Part model, mm, in its own coordinate system. A direction names the side the tool comes from. Give positions to 0.01 mm unless a question says otherwise; leave off trailing zeros. Loops run counter-clockwise (first coordinate to the right, second up) from the corner with the lowest first, then second, coordinate; pieces in that order, holes last. Notation, with made-up numbers: (48, 52) -> (59, 52) arc R25 cw to (59, 91) -> close; hole circle Ø4 at (25, 71). An arc over 180 degrees is marked (long way). One line per question, with ' | ' between items.
```python
from build123d import *

# Parameters (mm, degrees)
SKETCH1_R           = 3.935
EXTRUDE1_DEPTH      = 2
SKETCH2_R           = 2.7125
EXTRUDE2_DEPTH      = 1.4
SKETCH5_OUTSIDE_W   = 12.452
SKETCH5_OUTSIDE_H   = 12.452
SKETCH5_OUTSIDE_R   = 2.69
CUT_EXTRUDE1_DEPTH  = 0.35
CUT_EXTRUDE1_DRAFT  = 20
CHAMFER2_SIZE       = 0.127
SKETCH7_R           = 2
CUT_EXTRUDE3_DEPTH  = 7.521384056
BOSS_EXTRUDE1_DEPTH = 0.34
CIRPATTERN4_COUNT   = 30


with BuildPart() as part:
    # Sketch1 → Extrude1 (new body)
    with BuildSketch(Plane.XY):
        Circle(SKETCH1_R)
    extrude(amount=-EXTRUDE1_DEPTH)

    # Sketch2 → Extrude2 (add)
    with BuildSketch(Plane(origin=(0, 0, -2), x_dir=(-1, 0, 0), z_dir=(0, 0, -1))):
        with Locations(Location((0, 0, 0), (0, 0, 180))):
            Circle(SKETCH2_R)
    extrude(amount=EXTRUDE2_DEPTH)


with BuildPart() as cut_extrude1_tool:
    # Sketch5 outside → Cut-Extrude1 (with draft: the straight prism first)
    with BuildSketch(Plane(origin=(0, 0, -3.4), x_dir=(-1, 0, 0), z_dir=(0, 0, -1))):
        Rectangle(SKETCH5_OUTSIDE_W, SKETCH5_OUTSIDE_H)
        Circle(SKETCH5_OUTSIDE_R, mode=Mode.SUBTRACT)
    extrude(amount=-CUT_EXTRUDE1_DEPTH)
    # Cut-Extrude1: the draft: its side faces are tilted about the plane it starts from
    cut_extrude1_sides = [cut_extrude1_tool.faces().sort_by_distance(p)[0] for p in [
        (0, -6.226, -3.225),
        (-6.226, 0, -3.225),
        (0, 6.226, -3.225),
        (6.226, 0, -3.225),
        (2.69, 0, -3.225),
    ]]
    draft(cut_extrude1_sides, Plane(origin=(0, 0, -3.4), x_dir=(-1, 0, 0), z_dir=(0, 0, -1)), CUT_EXTRUDE1_DRAFT)


with BuildPart() as part_1:
    add(part.part)

    # Cut-Extrude1: cut by cut_extrude1_tool
    add(cut_extrude1_tool.part, mode=Mode.SUBTRACT)

    # Chamfer2
    chamfer2_edges = [part_1.edges().sort_by_distance(p)[0] for p in [
        (-3.935, 0, 0),
        (-3.935, 0, -2),
    ]]
    chamfer(chamfer2_edges, length=CHAMFER2_SIZE)

    # Sketch7 → Cut-Extrude3 (cut, through all)
    with BuildSketch(Plane.XY):
        Circle(SKETCH7_R)
    extrude(amount=-CUT_EXTRUDE3_DEPTH, mode=Mode.SUBTRACT)

    # Cut-Extrude6 cone 1 section (on through the dimple's axis) → Cut-Extrude6 (revolve, cut)
    with BuildSketch(Plane(origin=(0, 0, 0), x_dir=(0, -1, 0), z_dir=(1, 0, 0))):
        Polygon((0, 0), (2.0508, 0), (0, 2.0508), align=None)
    revolve(axis=Axis((0, 0, 0), (0, 0, -1)), mode=Mode.SUBTRACT)

    # Cut-Extrude7 cone 1 section (on through the dimple's axis) → Cut-Extrude7 (revolve, cut)
    with BuildSketch(Plane(origin=(0, 0, -3.4), x_dir=(0, 1, 0), z_dir=(1, 0, 0))):
        Polygon((0, 0), (2.0635, 0), (0, 2.0635), align=None)
    revolve(axis=Axis((0, 0, -3.4), (0, 0, 1)), mode=Mode.SUBTRACT)

    # Sketch16 → Boss-Extrude1 (add)
    with BuildSketch(Plane(origin=(0, 0, -2), x_dir=(-1, 0, 0), z_dir=(0, 0, -1))):
        with BuildLine():
            Line((0, 3.249), (-0.602777778, 2.644676767))
            ThreePointArc((-0.602777778, 2.644676767), (0, 2.7125), (0.602777778, 2.644676767))
            Line((0.602777778, 2.644676767), (0, 3.249))
        make_face()
    boss_extrude1 = extrude(amount=BOSS_EXTRUDE1_DEPTH)

    # CirPattern4: Boss-Extrude1 ×30 about axis
    cirpattern4_axis = Axis((0, 0, 0), (0, 0, 1))
    for i in range(1, CIRPATTERN4_COUNT):
        add(boss_extrude1.rotate(cirpattern4_axis, i * 360 / CIRPATTERN4_COUNT))


solid = part_1.part
```
1) Drill centre lines: line 1 (Y direction, x = 0, z = -0.9) (3 decimals); line 2 (Y direction, x = 0, z = -2.7); line 3 (Z direction, x = 3.25, y = -0.25). Where is each one in solid material? Low to high.
Found:
line 1: -3.935 to -2, 2 to 3.935 | line 2: -2.71 to -2, 2 to 2.71 | line 3: -2 to 0
2) Saw through at A-A (z = -2.7). Give the cut face in (x, y) (1 decimal), and give its area (3 significant figures).
Found:
outline: circle Ø5.4 at (0, 0); hole circle Ø4 at (0, 0) | area: 10.5 mm2
3) Saw through at B-B (z = -0.35). Give the cut face in (x, y) (3 decimals), and give its area (3 significant figures).
Found:
outline: circle Ø7.87 at (0, 0); hole circle Ø4 at (0, 0) | area: 36.1 mm2
4) Tool access for faces 1 (the flat face through (2, -2, 0)), 2 (the cylindrical face through (2.59, -0.81, -2.69)): list every direction of +Z, -Z, +X, -X, +Y, -Y with a clear straight run to the whole face (end or side of a thin tool).
Found:
face 1: +Z, +X, -X, +Y, -Y | face 2: -Z
